The model under review builds one solid part; all positions refer to its coordinate system, in mm. Face numbers are marked on the shaded views. Give positions to 0.01 mm unless a question says otherwise; leave off trailing zeros. Write each loop counter-clockwise with the first axis right and the second up, starting at its lowest first coordinate (ties: lowest second). Pieces come first, ordered by that corner, then holes.
Autodesk Inventor part; units mm, degrees
ref_plane "YZ Plane" through (0, 0, 0) normal (1, 0, 0) x (0, 1, 0)
ref_plane "XZ Plane" through (0, 0, 0) normal (0, 1, 0) x (-1, 0, 0)
ref_plane "XY Plane" through (0, 0, 0) normal (0, 0, 1) x (1, 0, 0)
sketch "Sketch1" plane through (0, 0, 0) normal (0, 0, 1) x (1, 0, 0)
  circle A0 centre (0, 0) radius 6
  circle A1 centre (0, 0) radius 4
  dimension "d0" = 12
  dimension "d1" = 8
extrude "Extrusion1" add sketch "Sketch1" along normal mid plane 4.6
fillet "Fillet2" radius 0.8 2 edges at (-6, 0, 2.3) (-6, 0, -2.3)
fillet "Fillet3" radius 0.6 2 edges at (-4, 0, 2.3) (-4, 0, -2.3)
properties part number "New_Tire"
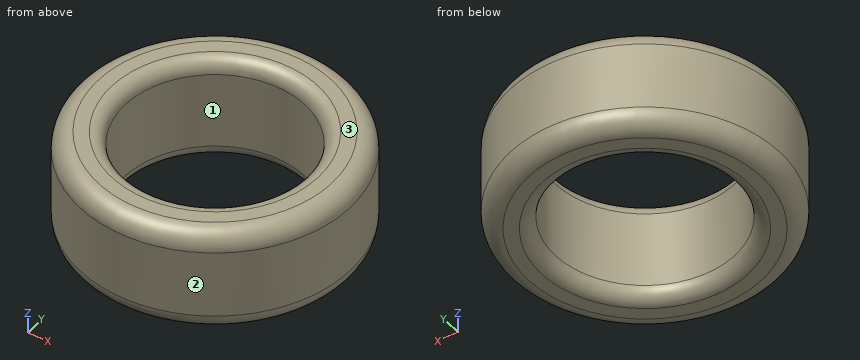
1) Insertion check: pin 1 (1 mm diameter, centred on x = -4, z = 2, fed in from +Y); pin 2 (1 mm diameter, centred on x = -3, z = -1, fed in from -Y). Each pin has a flat end and moves straight along its axis. Give the tip position at first contact, or say it passes through.
2) Consider section A-A, the plane y = 0. Give the boundary of the cut face in (x, z).
3) The part is to be moulded in two halves that separate along Y. For the marked faces 1, 2 and 3, say which applies: +Y half, -Y half, draft (parallel to the pull), parting line (faces both ways), or undercut.
4) To check wall thickness, follow probe 1 along Y at (x, z) = (0, 0.05); probe 2 along X at (y, z) = (-1, -0.3); probe 3 along X at (y, z) = (1.75, 1.65). State the ranges of each line that lie inside material, in increasing order.
5) Consider section C-C, the plane z = 0.65. Give the boundary of the cut face in (x, y).
Answer block:
1. pin 1: stops at y = 4.77
1. pin 2: stops at y = -5.45
2. outline: (-6, -1.5) arc R0.8 ccw to (-5.2, -2.3) - (-4.6, -2.3) arc R0.6 ccw to (-4, -1.7) - (-4, 1.7) arc R0.6 ccw to (-4.6, 2.3) - (-5.2, 2.3) arc R0.8 ccw to (-6, 1.5) - close; (4, -1.7) arc R0.6 ccw to (4.6, -2.3) - (5.2, -2.3) arc R0.8 ccw to (6, -1.5) - (6, 1.5) arc R0.8 ccw to (5.2, 2.3) - (4.6, 2.3) arc R0.6 ccw to (4, 1.7) - close
3. face 1: undercut
3. face 2: parting line
3. face 3: draft
4. probe 1: y = -6 to -4, 4 to 6
4. probe 2: x = -5.92 to -3.87, 3.87 to 5.92
4. probe 3: x = -5.72 to -3.6, 3.6 to 5.72
5. outline: circle Ø12 at (0, 0); hole circle Ø8 at (0, 0)
